Print and shaded views of the part. All mm, measured from the part's lowest x, y and z. A direction names the side the tool comes from. Coordinates: 2 decimals unless noted, no trailing zeros. Order: outer loops, then holes, each group sorted by start corner. A loop starts at its lowest first (then second) coordinate and runs counter-clockwise, first axis right, second up. Notation, with made-up numbers: M -17,89.25 L -10,89.25 A25 cw -10,115.25 Z; hole C 62,-23.75 d5. An arc over 180 degrees is marked long. One line per item, written item: value.
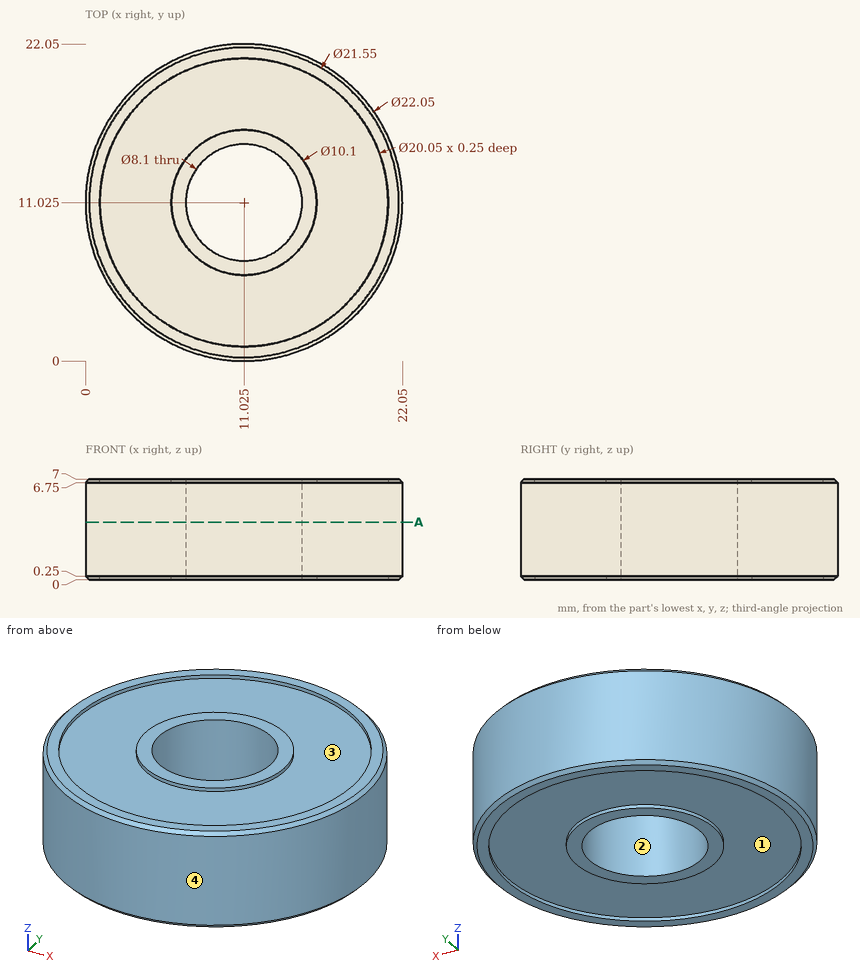
Q1. Pin check, flat tips, straight feed: pin 1 Ø1 at (x, y) = (10.5, 18.5) entering from +Z; pin 2 Ø4 at (x, z) = (6, 4) entering from +Y. Stop position of each tip, or through.
Recorded:
pin 1: stops at z = 6.75
pin 2: stops at y = 21.63
Q2. Drill centre lines: line 1 along Y through (x, z) = (8, 1); line 2 along Y through (x, z) = (11.25, 5); line 3 along Z through (x, y) = (17.5, 5.5). Where is each one in solid material? Low to high.
Recorded:
line 1: y = 0.42 to 8.33, 13.72 to 21.63
line 2: y = 0 to 6.98, 15.07 to 22.05
line 3: z = 0.25 to 6.75
Q3. Mould opens along Y. For the marked faces 3 and 4 say: released by +Y, released by -Y, zero draft, split by the parting line, or undercut.
Recorded:
face 3: undercut
face 4: split by the parting line
Q4. Slice it at A-A (z = 4). List the corners of the cut face in (x, y) (3 decimals), plus the area to 3 significant figures.
Recorded:
outline: C 11.025,11.025 d22.05; hole C 11.025,11.025 d8.1
area: 330 mm^2
Q5. Which spindle directions (+Z, -Z, +X, -X, +Y, -Y) get a long thin tool onto all of the face, cutting with end or side? Do the marked faces 1 and 2. Say none if no direction does.
Recorded:
face 1: -Z
face 2: +Z, -Z
